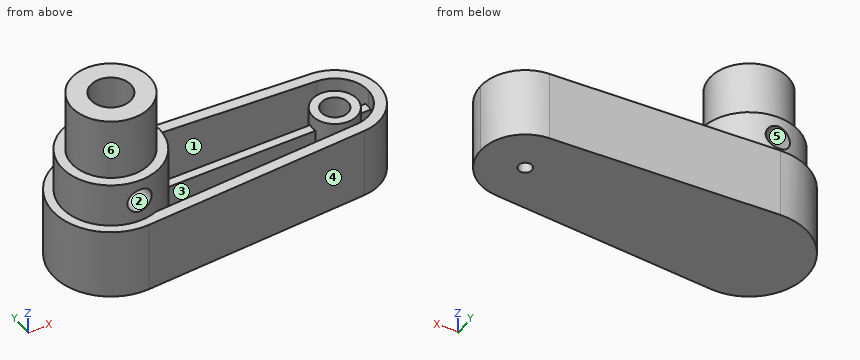
from build123d import *

# Parameters (mm, degrees)
F1_DEPTH        = 16
F2_T            = -2.5
F3_W            = 70
F3_H            = 2
F4_DEPTH        = 12
F6_R            = 11
F7_DEPTH        = 26
F5_R            = 5
F9_DEPTH        = 15
F8_R            = 8.75
F10_DEPTH       = 40
F12_D           = 9
F12_DEPTH       = 35
F12_TIP         = 2.7038727856
F13_R           = 2.7
F14_DEPTH       = 12.5
F16_D           = 3
F16_START       = 1
F16_CBORE_D     = 6
F16_CBORE_DEPTH = 5


with BuildPart() as f1:
    # F0 (on Top) → F1 (new body)
    with BuildSketch(Plane.XY):
        with BuildLine():
            ThreePointArc((0.78, -12.976578902), (9.4641428561, -8.9123509805), (13, 0))
            ThreePointArc((13, 0), (9.4641428561, 8.9123509805), (0.78, 12.976578902))
            ThreePointArc((0.78, 12.976578902), (-13, 0), (0.78, -12.976578902))
        make_face()
        with BuildLine():
            ThreePointArc((0.78, 12.976578902), (9.4641428561, 8.9123509805), (13, 0))
            ThreePointArc((13, 0), (9.4641428561, -8.9123509805), (0.78, -12.976578902))
            Line((0.78, -12.976578902), (50.6, -9.9819837708))
            ThreePointArc((50.6, -9.9819837708), (40, 0), (50.6, 9.9819837708))
            Line((50.6, 9.9819837708), (0.78, 12.976578902))
        make_face()
        with BuildLine():
            ThreePointArc((60, 0), (57.2801098893, 6.8556546004), (50.6, 9.9819837708))
            ThreePointArc((50.6, 9.9819837708), (40, 0), (50.6, -9.9819837708))
            ThreePointArc((50.6, -9.9819837708), (57.2801098893, -6.8556546004), (60, 0))
        make_face()
    extrude(amount=F1_DEPTH)

    # F2
    f2_openings = [f1.faces().sort_by_distance(p)[0] for p in [
        (21.977423, 0, 16),
    ]]
    offset(amount=F2_T, openings=f2_openings)

    # F3 (on Top) → F4 (join)
    with BuildSketch(Plane.XY):
        with Locations((23, 0)):
            Rectangle(F3_W, F3_H)
    extrude(amount=F4_DEPTH)

    # F6 (on Top) → F7 (join)
    with BuildSketch(Plane.XY):
        Circle(F6_R)
    extrude(amount=F7_DEPTH)

    # F5 (on Top) → F9 (join)
    with BuildSketch(Plane.XY):
        with Locations((50, 0)):
            Circle(F5_R)
    extrude(amount=F9_DEPTH)

    # F8 (on Top) → F10 (join)
    with BuildSketch(Plane.XY):
        Circle(F8_R)
    extrude(amount=F10_DEPTH)

    # F12
    with Locations(Plane.XY.offset(40)):
        with Locations((0, 0)):
            Hole(F12_D / 2, depth=F12_DEPTH)
            with Locations((0, 0, -(F12_DEPTH + F12_TIP / 2))):  # 118° drill point
                Cone(0, F12_D / 2, F12_TIP, mode=Mode.SUBTRACT)

    # F13 (on Front) → F14 (cut, symmetric)
    with BuildSketch(Plane.XZ):
        with Locations((0, 21)):
            Circle(F13_R)
    extrude(amount=F14_DEPTH, both=True, mode=Mode.SUBTRACT)

    # F16 (through all)
    # its depths count from where the whole tool has entered the part; down to there all is cleared
    with Locations(Plane.XY.offset(16).offset(-F16_START)):
        with Locations((50, 0)):
            CounterBoreHole(F16_D / 2, F16_CBORE_D / 2, F16_CBORE_DEPTH)


solid = f1.part
For this review, take the finished solid that the model builds, in its own axes (mm). Face numbers are marked on the shaded views. A direction names the side the tool comes from. Round coordinates to 2 decimals unless told otherwise and drop trailing zeros. Loops run counter-clockwise (first coordinate to the right, second up) from the corner with the lowest first, then second, coordinate; pieces in that order, holes last. Notation, with made-up numbers: (-15.5, 16) - (37.5, 16) arc R25 ccw to (37.5, 43) - close; hole circle Ø4 at (-23, 20). An arc over 180 degrees is marked (long way). One line per item, written item: value. Start each with the question number.
Item 1: Take a section at B-B (x = 36.5). Give the boundary of the cut face in (y, z) (3 decimals).
Item 2: Take a section at C-C (z = 31.5). Give the boundary of the cut face in (x, y), plus the area to 3 significant figures.
Item 3: The part is to be moulded in two halves that separate along X. For the marked faces 3, 4, 5 and 6, say which applies: +X half, -X half, draft (parallel to the pull), parting line (faces both ways), or undercut.
Item 4: Take a section at A-A (z = 13). Give the boundary of the cut face in (x, y), plus the area to 3 significant figures.
Item 5: Clearance check with flat-ended pins moving along their axes: pin 1 Ø5 at (x, y) = (28.5, -8.5) entering from +Z; pin 2 Ø3 at (x, y) = (30.5, 4.5) entering from +Z; pin 3 Ø10.5 at (x, z) = (30.5, 9.5) entering from -Y. State where each tip first meets the part, or that it passes through.
Item 6: For the marked faces 1 and 2, list the 3-axis set-ups (+Z, -Z, +X, -X, +Y, -Y) from which the entire face can be reached by the end or side of a thin tool; tool diameter is ignored.
Item 7: For L1, parallel to Z at x = 0, y = -7; L2, parallel to X at y = 2, z = 14.5; L3, parallel to Y at x = 50, z = 3, list the stretches that pass through material, from the lowest coordinate up.
Item 8: Take a section at D-D (z = 21). Give the boundary of the cut face in (x, y).
Answer below:
1. outline: (-10.83, 0) - (10.83, 0) - (10.83, 16) - (8.325, 16) - (8.325, 2.5) - (1, 2.5) - (1, 12) - (-1, 12) - (-1, 2.5) - (-8.325, 2.5) - (-8.325, 16) - (-10.83, 16) - close
2. outline: circle Ø17.5 at (0, 0); hole circle Ø9 at (0, 0)
2. area: 177 mm2
3. face 3: undercut
3. face 4: +X half
3. face 5: undercut
3. face 6: parting line
4. outline: (0.78, -12.98) - (50.6, -9.98) arc R10 ccw to (50.6, 9.98) - (0.78, 12.98) arc R13 ccw (long way) to start; circle Ø10 at (50, 0); hole circle Ø9 at (0, 0); hole (3.9, -10.28) - (50.45, -7.49) arc R7.5 ccw to (50.45, 7.49) - (3.9, 10.28) arc R11 cw to start; hole circle Ø6 at (50, 0)
4. area: 759 mm2
5. pin 1: stops at z = 16
5. pin 2: stops at z = 2.5
5. pin 3: stops at y = -11.51
6. face 1: +Z
6. face 2: +Y, -Y
7. L1: z = 0 to 18.3, 23.7 to 40
7. L2: x = -12.85 to -4.03, 4.03 to 10.82, 45.42 to 47.76, 52.24 to 54.58, 57.23 to 59.8
7. L3: y = -10.02 to -7.51, -5 to -1.5, 1.5 to 5, 7.51 to 10.02
8. outline: (-2.7, -10.66) - (-2.7, -3.6) arc R4.5 cw to (-2.7, 3.6) - (-2.7, 10.66) arc R11 ccw to start; (2.7, -10.66) arc R11 ccw to (2.7, 10.66) - (2.7, 3.6) arc R4.5 cw to (2.7, -3.6) - close
